Can you work these out from the model? Positions are in its coordinate system, mm. Face numbers are marked on the shaded views. A direction names the side the tool comes from. Round coordinates to 2 decimals unless told otherwise and drop trailing zeros. Loops run counter-clockwise (first coordinate to the right, second up) from the corner with the lowest first, then second, coordinate; pieces in that order, holes last. Notation, with made-up numbers: M 80,35.5 L 138,35.5 A14 ccw 138,59.5 Z; hole C 60.25,4.5 d6. An arc over 180 degrees is marked long. Answer as CSV lines item,"result".
from build123d import *

# Parameters (mm, degrees)
SKETCH1_W           = 50
SKETCH1_H           = 50
BOSS_EXTRUDE1_DEPTH = 10
SHELL1_T            = -2.5
SKETCH5_W           = 6
SKETCH5_H           = 6
BOSS_EXTRUDE3_DEPTH = 7.5
SKETCH9_R           = 3
CUT_EXTRUDE1_DEPTH  = 37.742346142
SKETCH15_W          = 4
SKETCH15_H          = 4
BOSS_EXTRUDE5_DEPTH = 4
M1_6_TAPPED_HOLE2_D = 1.25


with BuildPart() as part:
    # Sketch1 → Boss-Extrude1 (new body)
    with BuildSketch(Plane(origin=(0, 0, 0), x_dir=(1, 0, 0), z_dir=(0, 1, 0))):
        Rectangle(SKETCH1_W, SKETCH1_H)
    extrude(amount=BOSS_EXTRUDE1_DEPTH)

    # Shell1
    shell1_openings = [part.faces().sort_by_distance(p)[0] for p in [
        (0, 10, 0),
    ]]
    offset(amount=SHELL1_T, openings=shell1_openings, kind=Kind.INTERSECTION)

    # Sketch5 → Boss-Extrude3 (add)
    with BuildSketch(Plane(origin=(0, 2.5, 0), x_dir=(1, 0, 0), z_dir=(0, 1, 0))):
        with Locations((0, -19.5)):
            Rectangle(SKETCH5_W, SKETCH5_H)
    boss_extrude3 = extrude(amount=BOSS_EXTRUDE3_DEPTH)

    # Sketch8 → CSK SLOT for M1.6 Countersunk Flat Head Screw1 (revolve, cut)
    with BuildSketch(Plane(origin=(0, 0, 20.5), x_dir=(0, 0, -1), z_dir=(1, 0, 0))):
        Polygon((0, 0), (0, 10), (0.9, 10), (0.9, 9.4), (1.8, 8.5), (1.8, 0), align=None)
    csk_slot_for_m1_6_countersunk_flat_head = revolve(axis=Axis((0, -6.35, 20.5), (0, 1, 0)), mode=Mode.SUBTRACT)

    # Mirror1: Boss-Extrude3, CSK SLOT for M1.6 Countersunk Flat Head Screw1 across plane
    add(boss_extrude3.mirror(Plane.XY))
    add(csk_slot_for_m1_6_countersunk_flat_head.mirror(Plane.XY), mode=Mode.SUBTRACT)

    # Sketch9 → Cut-Extrude1 (cut, through all)
    with BuildSketch(Plane.XZ):
        with Locations(Location((0, 0, 0), (0, 0, 270))):
            Circle(SKETCH9_R)
    extrude(amount=-CUT_EXTRUDE1_DEPTH, mode=Mode.SUBTRACT)

    # Sketch15 → Boss-Extrude5 (add)
    with BuildSketch(Plane(origin=(0, 2.5, 0), x_dir=(1, 0, 0), z_dir=(0, 1, 0))):
        with Locations((-6.5, 0)):
            Rectangle(SKETCH15_W, SKETCH15_H)
        with Locations((6.5, 0)):
            Rectangle(SKETCH15_W, SKETCH15_H)
    extrude(amount=BOSS_EXTRUDE5_DEPTH)

    # M1.6 Tapped Hole2 (through all)
    with Locations(Plane(origin=(0, 0, 0), x_dir=(-1, 0, 0), z_dir=(0, -1, 0))):
        with Locations((-6.5, 0), (6.5, 0)):
            Hole(M1_6_TAPPED_HOLE2_D / 2)


solid = part.part
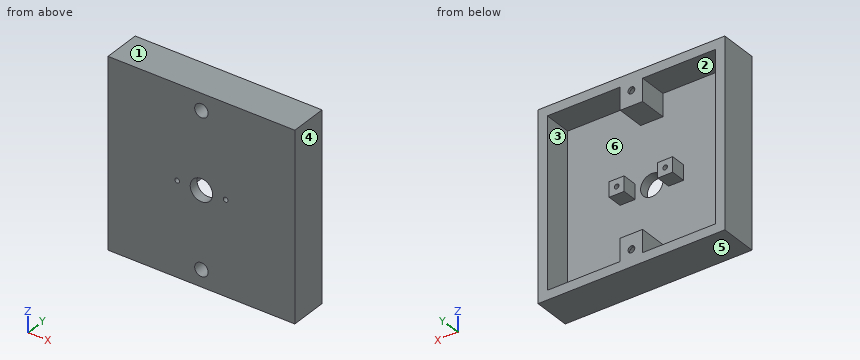
Item 1: If we section it at C-C on z = -20.5: Write out the boundary of the cut face in (x, y), then the cut area to 3 significant figures.
Output:
outline,"M -25,0 L -1.8,0 L -1.8,8.5 L -0.9,9.4 L -0.9,10 L -3,10 L -3,2.5 L -22.5,2.5 L -22.5,10 L -25,10 Z; M 0.9,9.4 L 1.8,8.5 L 1.8,0 L 25,0 L 25,10 L 22.5,10 L 22.5,2.5 L 3,2.5 L 3,10 L 0.9,10 Z"
area,"173 mm2"
Item 2: We'd pull the mould along X, two halves only. Please class the marked faces 1, 2, 3 and 4: released by +X, released by -X, zero draft, split by the parting line, or undercut.
Output:
face 1,"zero draft"
face 2,"undercut"
face 3,"undercut"
face 4,"released by +X"
Item 3: If I drill on line 1 along Z through (x, y) = (0, 9.75); line 2 along X through (y, z) = (6.25, 18); line 3 along Z through (x, y) = (0, 5), over which ranges is the centre line in solid material (lowest first)? Write a range as from..to.
Output:
line 1,"z = -25..-21.4, -19.6..-16.5, 16.5..19.6, 21.4..25"
line 2,"x = -25..-22.5, -3..3, 22.5..25"
line 3,"z = -25..-22.3, -18.7..-16.5, 16.5..18.7, 22.3..25"
Item 4: If we section it at D-D on z = 0: Write out the boundary of the cut face in (x, y) (3 decimals), then the cut area to 3 significant figures.
Output:
outline,"M -25,0 L -7.125,0 L -7.125,6.5 L -8.5,6.5 L -8.5,2.5 L -22.5,2.5 L -22.5,10 L -25,10 Z; M -5.875,0 L -3,0 L -3,2.5 L -4.5,2.5 L -4.5,6.5 L -5.875,6.5 Z; M 3,0 L 5.875,0 L 5.875,6.5 L 4.5,6.5 L 4.5,2.5 L 3,2.5 Z; M 7.125,0 L 25,0 L 25,10 L 22.5,10 L 22.5,2.5 L 8.5,2.5 L 8.5,6.5 L 7.125,6.5 Z"
area,"163 mm2"
Item 5: If we section it at A-A on y = 5: Write out the boundary of the cut face in (x, z) (3 decimals), then the cut area to 3 significant figures.
Output:
outline,"M -25,-25 L 25,-25 L 25,25 L -25,25 Z; M -8.5,-2 L -4.5,-2 L -4.5,2 L -8.5,2 Z; M 4.5,-2 L 8.5,-2 L 8.5,2 L 4.5,2 Z; hole M -22.5,-22.5 L -3,-22.5 L -3,-16.5 L 3,-16.5 L 3,-22.5 L 22.5,-22.5 L 22.5,22.5 L 3,22.5 L 3,16.5 L -3,16.5 L -3,22.5 L -22.5,22.5 Z; hole C -6.5,0 d1.25; hole C 0,-20.5 d3.6; hole C 0,20.5 d3.6; hole C 6.5,0 d1.25"
area,"556 mm2"
Item 6: Will these pins go through, and if not, where does the flat tip stop? pin 1 (2 mm diameter, centred on x = 6, z = -1, fed in from +Y); pin 2 (6 mm diameter, centred on x = 0, z = 20.5, fed in from +Y); pin 3 (8 mm diameter, centred on x = 0, z = 0, fed in from +Y).
Output:
pin 1,"stops at y = 6.5"
pin 2,"stops at y = 10"
pin 3,"stops at y = 2.5"
Item 7: If we section it at B-B on x = 0: Write out the boundary of the cut face in (y, z).
Output:
outline,"M 0,-25 L 10,-25 L 10,-21.4 L 9.4,-21.4 L 8.5,-22.3 L 0,-22.3 Z; M 0,-18.7 L 8.5,-18.7 L 9.4,-19.6 L 10,-19.6 L 10,-16.5 L 2.5,-16.5 L 2.5,-3 L 0,-3 Z; M 0,3 L 2.5,3 L 2.5,16.5 L 10,16.5 L 10,19.6 L 9.4,19.6 L 8.5,18.7 L 0,18.7 Z; M 0,22.3 L 8.5,22.3 L 9.4,21.4 L 10,21.4 L 10,25 L 0,25 Z"
Item 8: On a 3-axis mill with a long thin cutter (end or side, diameter ignored), from which of +Z, -Z, +X, -X, +Y, -Y can I reach the whole of each face in a straight line? I mean the marked faces 5 and 6. Say none if no direction works.
Output:
face 5,"-Z, +X, -X, +Y, -Y"
face 6,"+Y"
